Input: part model. Units: mm. Frame: model coordinates. A direction names the side the tool comes from. Give positions to 0.01 mm unless a question says otherwise; leave off trailing zeros. Loops run counter-clockwise (first coordinate to the right, second up) from the corner with the lowest first, then second, coordinate; pieces in that order, holes last. Notation, with made-up numbers: (59, 63.5) -> (112, 63.5) arc R10 ccw to (112, 67.5) -> close; hole circle Ø7 at (5.5, 46.5). An arc over 180 degrees is marked (long way). Use CSV: the item, a comma, the result in double quotes.
```python
from build123d import *

# Parameters (mm, degrees)
ESBO_O2_W                   = 144.687309412
ESBO_O2_H                   = 85.02541091
RESSALTO_EXTRUS_O2_DEPTH    = 5
RESSALTO_EXTRUS_O7_DEPTH    = 25
CORTE_EXTRUS_O11_DEPTH      = 164.107898205
CORTE_EXTRUS_O11_DEPTH_BACK = 164.107898205
ESBO_O16_W                  = 71.463749888
ESBO_O16_H                  = 7.00897528


with BuildPart() as part:
    # Esboço2 → Ressalto-extrusão2 (new, symmetric)
    with BuildSketch(Plane.XY):
        with Locations((-17.293303914, 0.144110866)):
            Rectangle(ESBO_O2_W, ESBO_O2_H)
    extrude(amount=RESSALTO_EXTRUS_O2_DEPTH, both=True)

    # Esboço4 → Ressalto-extrusão7 (add)
    with BuildSketch(Plane(origin=(0, 42.656816321, 0), x_dir=(1, 0, 0), z_dir=(0, 1, 0))):
        with BuildLine():
            Line((-66.189068435, 5), (-66.189068435, 71.35749318))
            ThreePointArc((-66.189068435, 71.35749318), (-31.056742356, 106.489819259), (4.075583724, 71.35749318))
            Line((4.075583724, 71.35749318), (4.075583724, 5))
            Line((4.075583724, 5), (-66.189068435, 5))
        make_face()
    extrude(amount=-RESSALTO_EXTRUS_O7_DEPTH)

    # Esboço13 → Rebaixo para parafuso de cabeça sextavada de M101 (revolve, cut)
    with BuildSketch(Plane(origin=(-32.523283398, 42.656816321, -64.100430101), x_dir=(0, 0, 1), z_dir=(1, 0, 0))):
        Polygon((0, 0), (0, 85.025410909), (5.5, 85.025410909), (5.5, 6.85), (10.74, 6.85), (10.74, 0.025), (10.765, 0), align=None)
    revolve(axis=Axis((-32.523283398, 49.006816321, -64.100430101), (0, -1, 0)), mode=Mode.SUBTRACT)

    # Esboço16 → Corte-extrusão11 (cut, two sides: drawn at the far end of the back side and taken through both)
    with BuildSketch(Plane(origin=(0, 42.656816321, 0), x_dir=(1, 0, 0), z_dir=(0, 1, 0)).offset(-CORTE_EXTRUS_O11_DEPTH_BACK)):
        with Locations((-30.531670696, -1.49551236)):
            Rectangle(ESBO_O16_W, ESBO_O16_H)
    extrude(amount=CORTE_EXTRUS_O11_DEPTH + CORTE_EXTRUS_O11_DEPTH_BACK, mode=Mode.SUBTRACT)


solid = part.part
```
1) Section query A-A (y = 28). Return loops of the section in (x, z).
From the geometry:
outline,"(-89.64, -5) -> (-66.19, -5) -> (-66.19, -71.36) arc R35.13 ccw to (4.08, -71.36) -> (4.08, -5) -> (55.05, -5) -> (55.05, 5) -> (5.2, 5) -> (5.2, -2.01) -> (-66.26, -2.01) -> (-66.26, 5) -> (-89.64, 5) -> close; hole circle Ø11 at (-32.52, -64.1)"
2) Ray query, line 1 (Y direction, x = -22.5, z = -15); line 2 (Z direction, x = -59.5, y = 10); line 3 (Z direction, x = 15, y = 24). Return the intervals inside material, ascending.
From the geometry:
line 1,"y = 17.66 to 42.66"
line 2,"z = -5 to -2.01"
line 3,"z = -5 to 5"
3) Section query D-D (z = -24). Return loops of the section in (x, y).
From the geometry:
outline,"(-66.19, 17.66) -> (4.08, 17.66) -> (4.08, 42.66) -> (-66.19, 42.66) -> close"
4) Mould query, pull axis X, two halves, no side actions, for faces 1 (the flat face through (-66.264, 0, 2)), 2 (the flat face through (-66.189, 30, -38)), 3 (the flat face through (4.076, 30, -39)). Classes: pulls with the +X half, pulls with the -X half, needs draft (parallel to the pull), parting line crosses it, or undercut.
From the geometry:
face 1,"undercut"
face 2,"pulls with the -X half"
face 3,"pulls with the +X half"
5) Reachability of faces 4 (the flat face through (-31, 0, -2.009)), 5 (the flat face through (-31, 17.657, -56)), 6 (the flat face through (-35, 35.807, -59)) from +Z, -Z, +X, -X, +Y, -Y: full face, straight path, thin tool, end or side. Return the list, or none.
From the geometry:
face 4,"+Z, +Y, -Y"
face 5,"-Z, +X, -X, -Y"
face 6,"+Y"
6) Contact query for flat-ended pins moving along their axis: pin 1 (6.5 mm diameter, centred on x = -34.5, z = -68, fed in from +Y); pin 2 (10 mm diameter, centred on x = -32.52, z = -64.1, fed in from -Y); pin 3 (12 mm diameter, centred on y = 17.5, z = -21.5, fed in from -X); pin 4 (20 mm diameter, centred on y = 29, z = -32.5, fed in from +X). Output: stop coordinate, or through.
From the geometry:
pin 1,"stops at y = 35.81"
pin 2,"passes through"
pin 3,"stops at x = -66.19"
pin 4,"stops at x = 4.08"
7) Section query B-B (y = -13). Return loops of the section in (x, z).
From the geometry:
outline,"(-89.64, -5) -> (55.05, -5) -> (55.05, 5) -> (5.2, 5) -> (5.2, -2.01) -> (-66.26, -2.01) -> (-66.26, 5) -> (-89.64, 5) -> close"
8) Section query C-C (x = -50.5). Return loops of the section in (y, z).
From the geometry:
outline,"(-42.37, -5) -> (17.66, -5) -> (17.66, -100.62) -> (42.66, -100.62) -> (42.66, -2.01) -> (-42.37, -2.01) -> close"
